Input: part model. Units: mm. Frame: model coordinates. Coordinates: 2 decimals unless noted, no trailing zeros. Loops run counter-clockwise (first coordinate to the right, second up) from the corner with the lowest first, then second, coordinate; pieces in that order, holes last. Notation, with made-up numbers: (-22.5, 53.5) - (6.5, 53.5) arc R13 ccw to (6.5, 71.5) - close; hole circle Ø8 at (-36.5, -26). An arc over 180 degrees is marked (long way). Use one line per item in the form item = value.
from build123d import *

# Parameters (mm, degrees)
F0_W     = 90
F0_H     = 100
F1_DEPTH = 20
F2_D     = 6.5
F3_D     = 5
F4_D     = 3.5
F6_D     = 3.6
F6_DEPTH = 16
F6_TIP   = 1.0815491142
F8_D     = 3.6
F8_DEPTH = 16
F8_TIP   = 1.0815491142


with BuildPart() as f1:
    # F0 (on Top) → F1 (new body)
    with BuildSketch(Plane.XY):
        Rectangle(F0_W, F0_H)
    extrude(amount=-F1_DEPTH)

    # F2 (through all)
    with Locations(Plane.XY):
        with Locations((-35, 35), (-35, 0), (-35, -35)):
            Hole(F2_D / 2)

    # F3 (through all)
    with Locations(Plane.XY):
        with Locations((0, 35), (0, 0), (0, -35)):
            Hole(F3_D / 2)

    # F4 (through all)
    with Locations(Plane.XY):
        with Locations((35, 35), (35, 0), (35, -35)):
            Hole(F4_D / 2)

    # F6
    with Locations(Plane(origin=(-45, 0, 0), x_dir=(0, -1, 0), z_dir=(-1, 0, 0))):
        with Locations((-25, -10), (25, -10)):
            Hole(F6_D / 2, depth=F6_DEPTH)
            with Locations((0, 0, -(F6_DEPTH + F6_TIP / 2))):  # 118° drill point
                Cone(0, F6_D / 2, F6_TIP, mode=Mode.SUBTRACT)

    # F8
    with Locations(Plane.YZ.offset(45)):
        with Locations((-25, -10), (25, -10)):
            Hole(F8_D / 2, depth=F8_DEPTH)
            with Locations((0, 0, -(F8_DEPTH + F8_TIP / 2))):  # 118° drill point
                Cone(0, F8_D / 2, F8_TIP, mode=Mode.SUBTRACT)


solid = f1.part
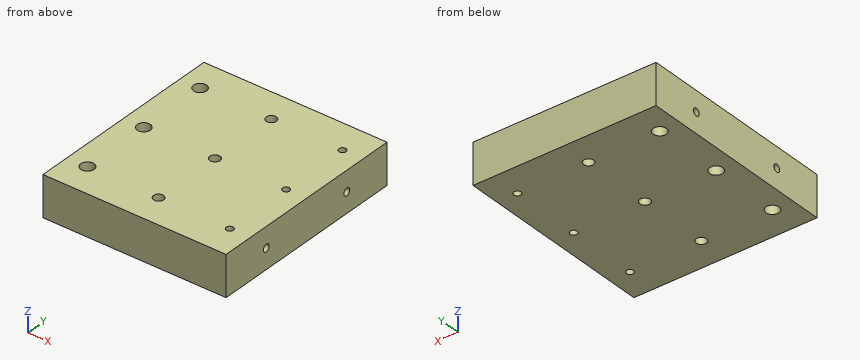
Q1. Cut plane C-C, the plane z = -2.25. Give the number of separate pieces and of enclosed holes in the cut face, then the cut area to 3 significant figures.
Check values:
separate_pieces = 1
enclosed_holes = 9
area = 8,810 mm²
Q2. Ray query, line 1 along Y through (x, z) = (-35, -15.5); line 2 along Y through (x, z) = (36.5, -5.75); line 3 along Z through (x, y) = (36, -25). Return the intervals inside material, ascending. Write a range as [from, to].
Check values:
line_1 = [-50, -38.25], [-31.75, -3.25], [3.25, 31.75], [38.25, 50]
line_2 = [-50, -35.9], [-34.1, -0.9], [0.9, 34.1], [35.9, 50]
line_3 = [-20, -11.8], [-8.2, 0]
Q3. First-contact query: P1, Ø4, axis at x = 35, y = 0, coming from the -Z side; P2, Ø3, axis at y = -25, z = -10, coming from the +X side. Flat tips, straight axial feed; report the tip coordinate or a pass-through.
Check values:
P1 = -20
P2 = 28.82
Q4. Cut plane B-B, the plane y = -35. Return loops of the section in (x, z), then the cut area to 3 significant figures.
Check values:
outline = (-45, -20) - (-38.25, -20) - (-38.25, 0) - (-45, 0) - close; (-31.75, -20) - (-2.5, -20) - (-2.5, 0) - (-31.75, 0) - close; (2.5, -20) - (33.25, -20) - (33.25, 0) - (2.5, 0) - close; (36.75, -20) - (45, -20) - (45, 0) - (36.75, 0) - close
area = 1,500 mm²
Q5. Cut plane A-A, the plane x = -35. Return loops of the section in (y, z), then the cut area to 3 significant figures.
Check values:
outline = (-50, -20) - (-38.25, -20) - (-38.25, 0) - (-50, 0) - close; (-31.75, -20) - (-3.25, -20) - (-3.25, 0) - (-31.75, 0) - close; (3.25, -20) - (31.75, -20) - (31.75, 0) - (3.25, 0) - close; (38.25, -20) - (50, -20) - (50, 0) - (38.25, 0) - close; hole circle Ø3.6 at (-25, -10); hole circle Ø3.6 at (25, -10)
area = 1,590 mm²
Q6. Cut plane D-D, the plane x = 0. Return loops of the section in (y, z), then the cut area to 3 significant figures.
Check values:
outline = (-50, -20) - (-37.5, -20) - (-37.5, 0) - (-50, 0) - close; (-32.5, -20) - (-2.5, -20) - (-2.5, 0) - (-32.5, 0) - close; (2.5, -20) - (32.5, -20) - (32.5, 0) - (2.5, 0) - close; (37.5, -20) - (50, -20) - (50, 0) - (37.5, 0) - close
area = 1,700 mm²
